```python
from build123d import *

# Parameters (mm, degrees)
CROQUIS1_R                   = 7
SALIENTE_EXTRUIR1_DEPTH      = 15
CROQUIS2_R                   = 10
SALIENTE_EXTRUIR2_DEPTH      = 50
SALIENTE_EXTRUIR3_DEPTH      = 30
SALIENTE_EXTRUIR3_DEPTH_BACK = 6
CROQUIS3_W                   = 10
CROQUIS3_H                   = 15
CHAFL_N1_SIZE                = 30
CHAFL_N1_SIZE_2              = 23.438568795
CROQUIS4_R                   = 6
CORTAR_EXTRUIR1_DEPTH        = 20


with BuildPart() as part:
    # Croquis1 → Saliente-Extruir1 (new body)
    with BuildSketch(Plane(origin=(0, 0, 0), x_dir=(1, 0, 0), z_dir=(0, 1, 0))):
        with Locations(Location((0, 0, 0), (0, 0, 270))):
            Circle(CROQUIS1_R)
    extrude(amount=SALIENTE_EXTRUIR1_DEPTH)

    # Croquis2 → Saliente-Extruir2 (add)
    with BuildSketch(Plane(origin=(0, 15, 0), x_dir=(1, 0, 0), z_dir=(0, 1, 0))):
        with Locations(Location((0, 0, 0), (0, 0, 270))):
            Circle(CROQUIS2_R)
    extrude(amount=SALIENTE_EXTRUIR2_DEPTH)

    # Croquis3 → Saliente-Extruir3 (add, two sides: drawn at the far end of the back side and taken through both)
    with BuildSketch(Plane.XY.offset(10).offset(-SALIENTE_EXTRUIR3_DEPTH_BACK)):
        with Locations((3, 53.5)):
            Rectangle(CROQUIS3_W, CROQUIS3_H)
    extrude(amount=SALIENTE_EXTRUIR3_DEPTH + SALIENTE_EXTRUIR3_DEPTH_BACK)

    # Chaflán1
    # the kernel refuses this chamfer: 30, 23.438568795 mm, written as the material it takes off along each edge
    with BuildSketch(Plane(origin=(85.38607652, 61, 40), x_dir=(0, 0.023867141339117135, -0.9997151392093142), z_dir=(-1, 0, 0))) as chafl_n1_piece_1_section:
        Polygon((CHAFL_N1_SIZE * 0.999715139209, CHAFL_N1_SIZE * 0.0238671413391), (-CHAFL_N1_SIZE_2 * 0.0238671413393, CHAFL_N1_SIZE_2 * 0.999715139218), (0, 0), align=None)
    chafl_n1_piece_1 = extrude(amount=164.77215304, mode=Mode.PRIVATE)
    chafl_n1_piece_1 = chafl_n1_piece_1 - Plane(origin=(0, 53.349255428, 0), x_dir=(0, 0, 1), z_dir=(0, -1, 0)) * Cylinder(10, 450, mode=Mode.PRIVATE)
    add(chafl_n1_piece_1, mode=Mode.SUBTRACT)

    # Croquis4 → Cortar-Extruir1 (cut)
    with BuildSketch(Plane(origin=(0, 65, 0), x_dir=(1, 0, 0), z_dir=(0, 1, 0))):
        with Locations(Location((0, 0, 0), (0, 0, 270))):
            Circle(CROQUIS4_R)
    extrude(amount=-CORTAR_EXTRUIR1_DEPTH, mode=Mode.SUBTRACT)


solid = part.part
```
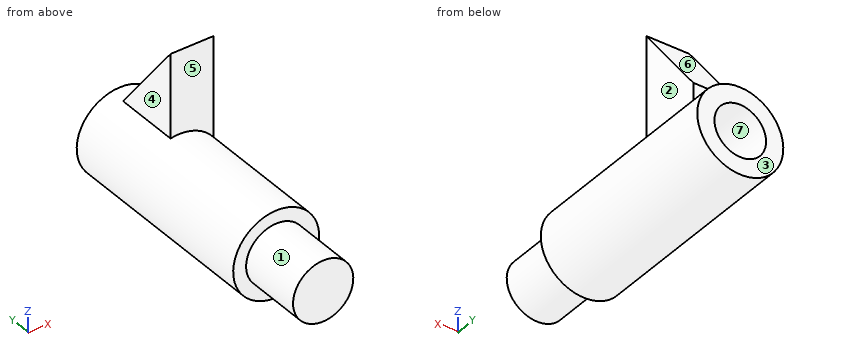
Geometry: final body of the model. Coordinates: model frame, mm. Face numbers are marked on the shaded views. A direction names the side the tool comes from. Round coordinates to 2 decimals unless told otherwise and drop trailing zeros. Order: outer loops, then holes, each group sorted by start corner. A loop starts at its lowest first (then second) coordinate and runs counter-clockwise, first axis right, second up. Notation, with made-up numbers: (-37, 62) - (-3, 62) arc R21 ccw to (-3, 78) - close; hole circle Ø1 at (88, -12). An arc over 180 degrees is marked (long way). Write item = value, one per line. Start each with the question number.
Q1. Access query for the marked faces 1, 2, 3 and 4. Directions: +Z, -Z, +X, -X, +Y, -Y. A direction counts if a zero-diameter tool reaches every point of the face in a straight line with its end or side. Return the directions, or none.
Q2. Pull-direction query (Z, two-part tool) for the marked faces 5, 6 and 7; classes: +Z half, -Z half, draft (parallel to the pull), parting line (faces both ways), or undercut.
Q3. Cut plane B-B on x = 1. Return the cut outline in (y, z).
Q4. Cut plane D-D on y = 51. Return the cut outline in (x, z).
Q5. Pin query (flat end, axial travel): pin 1 (2 mm diameter, centred on x = -4.5, z = -2, fed in from -Y); pin 2 (11 mm diameter, centred on x = 2, z = 14.5, fed in from -Y); pin 3 (12 mm diameter, centred on x = 1, y = 8, fed in from -Z); pin 4 (3 mm diameter, centred on x = 6, y = 22.5, fed in from +Z). Return the tip coordinate at first contact, or that it passes through.
Q6. Cut plane C-C on y = 44. Return the cut outline in (x, z).
Q7. Cut plane A-A on z = 0. Return the cut outline in (x, y), and give its area (3 significant figures).
Q8. Ray query, line 1 (X direction, y = 61, z = 0); line 2 (Y direction, x = 4.25, z = -3); line 3 (Z direction, x = 0.25, y = 42.5). Return the intervals inside material, ascending. Write a range as from..to.
Outcome:
q1.face_1 = -Y
q1.face_2 = +Z, +X, +Y, -Y
q1.face_3 = +Z, -Z, +X, -X, +Y
q1.face_4 = +Z, -X, +Y, -Y
q2.face_5 = draft
q2.face_6 = +Z half
q2.face_7 = undercut
q3.outline = (0, -6.93) - (15, -6.93) - (15, -9.95) - (65, -9.95) - (65, -5.92) - (45, -5.92) - (45, 5.92) - (65, 5.92) - (65, 9.95) - (61, 9.95) - (61, 10) - (46, 29.2) - (46, 9.95) - (15, 9.95) - (15, 6.93) - (0, 6.93) - close
q4.outline = (-2, 9.8) arc R10 ccw (long way) to (8, 6) - (8, 22.8) - (-2, 22.8) - close; hole circle Ø12 at (0, 0)
q5.pin_1 = 0
q5.pin_2 = 15
q5.pin_3 = -7
q5.pin_4 = 8.93
q6.outline = circle Ø20 at (0, 0)
q7.outline = (-10, 15) - (-7, 15) - (-7, 0) - (7, 0) - (7, 15) - (10, 15) - (10, 65) - (6, 65) - (6, 45) - (-6, 45) - (-6, 65) - (-10, 65) - close
q7.area = 970 mm^2
q8.line_1 = -10..-6, 6..10
q8.line_2 = 0..45
q8.line_3 = -10..10
